Input: part model. Units: mm. Frame: model coordinates. Face numbers are marked on the shaded views. A direction names the side the tool comes from. Give positions to 0.01 mm unless a question says otherwise; leave off trailing zeros. Write each loop counter-clockwise with the first axis right and the second up, starting at its lowest first coordinate (ties: lowest second). Pieces come first, ordered by that corner, then holes. Notation, with made-up numbers: (-14, 63) - (-8, 63) arc R22 cw to (-8, 75) - close; hole circle Ø6 at (73, 18.25). An arc over 180 degrees is marked (long way). Use a Markdown table: item, result. Add a question column.
1. Material intervals for probe 1 along Y at (x, z) = (-60, -6); probe 2 along X at (y, z) = (17, -4); probe 3 along Y at (x, z) = (-58, -3.25), sorted ascending.
2. Pin query (flat end, axial travel): pin 1 (2 mm diameter, centred on y = 19, z = -3.5, fed in from -X); pin 2 (4.5 mm diameter, centred on y = 20.5, z = -6.5, fed in from +X). Return the tip coordinate at first contact, or that it passes through.
3. Section query D-D, the plane y = 7.5. Return loops of the section in (x, z), plus the area to 3 significant figures.
4. Section query A-A, the plane z = -4. Return loops of the section in (x, y), plus the area to 3 significant figures.
5. Set-up query: the marked faces 1, 2 and 3. Return all of +Z, -Z, +X, -X, +Y, -Y with unobstructed straight access to the full face (end or side cutting, diameter ignored); none if empty.
6. Section query C-C, the plane y = 19.5. Return loops of the section in (x, z).
7. Section query B-B, the plane x = -60. Return loops of the section in (y, z), plus the area to 3 significant figures.
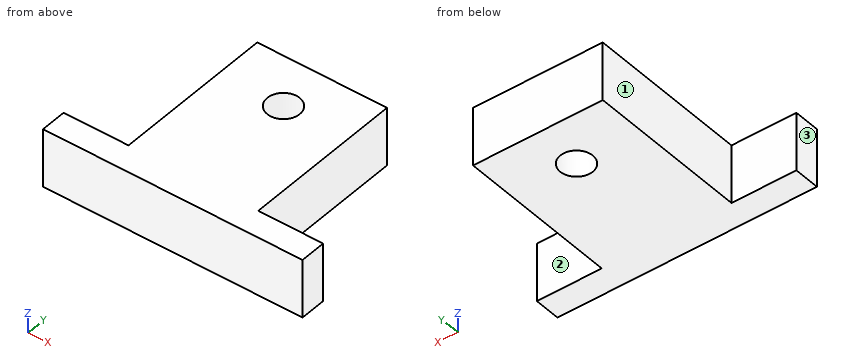
```python
from build123d import *

# Parameters (mm, degrees)
BOSS_EXTRU_2_DEPTH      = 9
ESQUISSE1_4_R           = 2.5
ENL_V_MAT_EXTRU_6_DEPTH = 86.568685861


with BuildPart() as part:
    # Esquisse1 → Boss.-Extru.2 (new body)
    with BuildSketch(Plane.XY):
        Polygon((-40, 0), (-80, 0), (-80, 4), (-70, 4), (-70, 29), (-50, 29), (-50, 4), (-40, 4), align=None)
    extrude(amount=-BOSS_EXTRU_2_DEPTH)

    # Esquisse1<4> → Enlèv. mat.-Extru.6 (cut, through all)
    with BuildSketch(Plane.XY):
        with Locations((-60, 21.5)):
            Circle(ESQUISSE1_4_R)
    extrude(amount=-ENL_V_MAT_EXTRU_6_DEPTH, mode=Mode.SUBTRACT)


solid = part.part
```
Result sheet:
| question | item | result |
|---|---|---|
| 1 | probe 1 | y = 0 to 19, 24 to 29 |
| 1 | probe 2 | x = -70 to -50 |
| 1 | probe 3 | y = 0 to 20, 23 to 29 |
| 2 | pin 1 | stops at x = -70 |
| 2 | pin 2 | stops at x = -50 |
| 3 | outline | (-70, -9) - (-50, -9) - (-50, 0) - (-70, 0) - close |
| 3 | area | 180 mm² |
| 4 | outline | (-80, 0) - (-40, 0) - (-40, 4) - (-50, 4) - (-50, 29) - (-70, 29) - (-70, 4) - (-80, 4) - close; hole circle Ø5 at (-60, 21.5) |
| 4 | area | 640 mm² |
| 5 | face 1 | +Z, -Z, -X, +Y |
| 5 | face 2 | +Z, -Z, +X, +Y |
| 5 | face 3 | +Z, -Z, -X, +Y, -Y |
| 6 | outline | (-70, -9) - (-61.5, -9) - (-61.5, 0) - (-70, 0) - close; (-58.5, -9) - (-50, -9) - (-50, 0) - (-58.5, 0) - close |
| 7 | outline | (0, -9) - (19, -9) - (19, 0) - (0, 0) - close; (24, -9) - (29, -9) - (29, 0) - (24, 0) - close |
| 7 | area | 216 mm² |
